Part model, mm, in its own coordinate system. A direction names the side the tool comes from. Round coordinates to 2 decimals unless told otherwise and drop trailing zeros. Write each loop counter-clockwise with the first axis right and the second up, starting at its lowest first coordinate (ties: lowest second). Pieces come first, ordered by that corner, then holes.
1) Flat gauge pins, fed straight in: pin 1 (6 mm diameter, centred on y = -0.5, z = 5.5, fed in from +X); pin 2 (6 mm diameter, centred on x = 3.5, z = 5, fed in from -Y); pin 3 (4.5 mm diameter, centred on x = 0, y = 8.5, fed in from -Z); pin 4 (6 mm diameter, centred on y = -4, z = -2.5, fed in from -X). Where does each tip first touch, or does it go through?
2) Saw through at D-D on y = 6.5. Write the cut outline in (x, z).
3) Pull direction Z, two halves, no side cores. Call faces 6 (the flat face through (0, 2, -12)), 7 (the flat face through (0, 10, -6)), 8 (the flat face through (0, 7, 0)): +Z half, -Z half, draft (parallel to the pull), parting line (faces both ways), or undercut.
4) Saw through at B-B on z = -6. Write the cut outline in (x, y).
5) Which spindle directions (+Z, -Z, +X, -X, +Y, -Y) get a long thin tool onto all of the face, cutting with end or side? Do faces 1 (the flat face through (0, -7, 0)), 2 (the cylindrical face through (0.325, -7.465, -7.464)), 3 (the flat face through (0, -2, 9)), 4 (the cylindrical face through (0.325, 7.465, -4.536)), 5 (the flat face through (-5, 2, 6.75)). Say none if no direction does.
6) Drill centre lines: L1, parallel to Z at x = 3.25, y = 6.5; L2, parallel to Y at x = 0, z = -5; L3, parallel to Y at x = 0, z = 3. Where is each one in solid material? Low to high.
7) Saw through at A-A on y = 0. Write the cut outline in (x, z).
Autodesk Inventor part; units mm, degrees
ref_plane "YZ Plane" through (0, 0, 0) normal (1, 0, 0) x (0, 1, 0)
ref_plane "XZ Plane" through (0, 0, 0) normal (0, 1, 0) x (-1, 0, 0)
ref_plane "XY Plane" through (0, 0, 0) normal (0, 0, 1) x (1, 0, 0)
sketch "Sketch1" plane through (0, 0, 0) normal (0, 0, 1) x (1, 0, 0)
  arc A0 (-8.9303, 4.5) -> (-8.9303, -4.5) centre (0, 0) ccw
  circle A1 centre (0, 0) radius 4.5 construction
  line L0 (-8.9303, 4.5) -> (8.9303, 4.5)
  line L1 (-8.9303, -4.5) -> (8.9303, -4.5)
  arc A2 (8.9303, 4.5) -> (-8.9303, 4.5) centre (0, 0) ccw
  arc A3 (8.9303, -4.5) -> (8.9303, 4.5) centre (0, 0) ccw
  arc A4 (-8.9303, -4.5) -> (8.9303, -4.5) centre (0, 0) ccw
  dimension "d0" = 20
  dimension "d1" = 9
extrude "Extrusion1" add sketch "Sketch1" against normal blind 12 contours L0 A3 L1 A0
extrude "Extrusion2" add sketch "Sketch1" along normal blind 9
sketch "Sketch2" plane through (0, 0, 0) normal (0, 1, 0) x (-1, 0, 0)
  circle A0 centre (0, -6) radius 1.5
  line L0 (0, 0) -> (0, -6) construction
  dimension "d6" = 3
  dimension "d7" = 6
extrude "Extrusion3" add sketch "Sketch2" along normal mid plane 20
sketch "Sketch3" plane through (0, 0, 0) normal (0, 1, 0) x (-1, 0, 0)
  line L0 (10, 9) -> (-10, 9) construction
  line L1 (8.9303, 0) -> (-8.9303, 0) construction
  line L2 (0, 9) -> (0, 0) construction
  line L3 (-8.9303, 0) -> (8.9303, 0) construction
  line L4 (0, 4.5) -> (-10, 4.5) construction
  line L5 (-10, 9) -> (-10, -12) construction
  line L6 (-5, 2.25) -> (-10, 2.25)
  line L7 (-10, 2.25) -> (-10, 6.75)
  line L8 (-10, 6.75) -> (-5, 6.75)
  line L9 (-5, 6.75) -> (-5, 2.25)
  line L10 (-5, 2.25) -> (-10, 6.75) construction
  line L11 (-10, 2.25) -> (-5, 6.75) construction
  point P0 (-7.5, 4.5)
  dimension "d10" = 4.5
  dimension "d11" = 10
revolve "Revolution1" cut sketch "Sketch3" angle 360 about axis through (0, 0, 9) along (0, 0, -1)
sketch "Sketch4" plane through (0, 0, 0) normal (0, 0, 1) x (1, 0, 0)
  circle A0 centre (0, 0) radius 1.6
  dimension "d22" = 3.2
extrude "Extrusion4" cut sketch "Sketch4" along normal through all both and the other way through all
chamfer "Chamfer1" [suppressed]
fillet "Fillet1" radius 0.5 2 edges at (1.5, -4.5, -6) (1.5, 4.5, -6)
properties part number "slider-1"
Completed:
1. pin 1: stops at x = 10
1. pin 2: stops at y = -9.94
1. pin 3: stops at z = -7.5
1. pin 4: stops at x = -9.95
2. outline: (-7.6, 0) - (7.6, 0) - (7.6, 2.25) - (-7.6, 2.25) - close; (-7.6, 6.75) - (7.6, 6.75) - (7.6, 9) - (-7.6, 9) - close; circle Ø3 at (0, -6)
3. face 6: -Z half
3. face 7: draft
3. face 8: undercut
4. outline: (-8.93, -4.5) - (-2, -4.5) arc R0.5 cw to (-1.5, -5) - (-1.5, -10) - (1.5, -10) - (1.5, -5) arc R0.5 cw to (2, -4.5) - (8.93, -4.5) arc R10 ccw to (8.93, 4.5) - (2, 4.5) arc R0.5 cw to (1.5, 5) - (1.5, 10) - (-1.5, 10) - (-1.5, 5) arc R0.5 cw to (-2, 4.5) - (-8.93, 4.5) arc R10 ccw to start; hole circle Ø3.2 at (0, 0)
5. face 1: +X, -X, -Y
5. face 2: -Y
5. face 3: +Z, +X, -X, +Y, -Y
5. face 4: +Y
5. face 5: none
6. L1: z = 0 to 2.25, 6.75 to 9
6. L2: y = -10 to -1.6, 1.6 to 10
6. L3: y = -5 to -1.6, 1.6 to 5
7. outline: (-10, -12) - (-1.6, -12) - (-1.6, 9) - (-10, 9) - (-10, 6.75) - (-5, 6.75) - (-5, 2.25) - (-10, 2.25) - close; (1.6, -12) - (10, -12) - (10, 2.25) - (5, 2.25) - (5, 6.75) - (10, 6.75) - (10, 9) - (1.6, 9) - close
